```python
from build123d import *

# Parameters (mm, degrees)
F0_W     = 66.04
F0_H     = 22
F1_DEPTH = 69.85
F2_R     = 5.08


with BuildPart() as f1:
    # F0 (on Top) → F1 (new body)
    with BuildSketch(Plane.XY):
        Rectangle(F0_W, F0_H)
        with BuildLine():
            ThreePointArc((-23.97354, 8.353052), (-14.017672, 7.055087), (-11.109783, -2.554711))
            ThreePointArc((-11.109783, -2.554711), (-10.464057, -8.085959), (-16.02646, -8.353052))
            ThreePointArc((-16.02646, -8.353052), (-25.982328, -7.055087), (-28.890217, 2.554711))
            ThreePointArc((-28.890217, 2.554711), (-29.535943, 8.085959), (-23.97354, 8.353052))
        make_face(mode=Mode.SUBTRACT)
        with BuildLine():
            ThreePointArc((3.97354, -8.353052), (-5.982328, -7.055087), (-8.890217, 2.554711))
            ThreePointArc((-8.890217, 2.554711), (-9.535943, 8.085959), (-3.97354, 8.353052))
            ThreePointArc((-3.97354, 8.353052), (5.982328, 7.055087), (8.890217, -2.554711))
            ThreePointArc((8.890217, -2.554711), (9.535943, -8.085959), (3.97354, -8.353052))
        make_face(mode=Mode.SUBTRACT)
        with BuildLine():
            ThreePointArc((16.02646, 8.353052), (25.982328, 7.055087), (28.890217, -2.554711))
            ThreePointArc((28.890217, -2.554711), (29.535943, -8.085959), (23.97354, -8.353052))
            ThreePointArc((23.97354, -8.353052), (14.017672, -7.055087), (11.109783, 2.554711))
            ThreePointArc((11.109783, 2.554711), (10.464057, 8.085959), (16.02646, 8.353052))
        make_face(mode=Mode.SUBTRACT)
    extrude(amount=F1_DEPTH)

    # F2
    f2_edges = [f1.edges().sort_by_distance(p)[0] for p in [
        (-33.02, 11, 34.925),
        (-33.02, -11, 34.925),
        (33.02, -11, 34.925),
        (33.02, 11, 34.925),
    ]]
    fillet(f2_edges, radius=F2_R)


solid = f1.part
```
CAD build for the part. Positions are in the model's coordinates, mm. Coordinates: 2 decimals unless noted, no trailing zeros. Order: outer loops, then holes, each group sorted by start corner. A loop starts at its lowest first (then second) coordinate and runs counter-clockwise, first axis right, second up. Notation, with made-up numbers: (59, 45.5) - (76, 45.5) arc R27 ccw to (76, 67.5) - close; hole circle Ø6 at (57, 11). An arc over 180 degrees is marked (long way). Use a Markdown table: item, result. Add a question column.
(1) Flat gauge pins, fed straight in: pin 1 (1.5 mm diameter, centred on y = 8, z = 60, fed in from -X); pin 2 (5 mm diameter, centred on x = -18, y = 6, fed in from -Z). Where does each tip first touch, or does it go through?
(2) Saw through at A-A (x = -19). Give the cut face in (y, z), then the cut area to 3 significant figures.
(3) Saw through at C-C (z = 35). Give the cut face in (x, y).
(4) Drill centre lines: line 1 along X through (y, z) = (0.5, 61); line 2 along X through (y, z) = (2.75, 60); line 3 along Y through (x, z) = (-20.5, 19). Where is each one in solid material? Low to high. Write a range as [from, to].
(5) Pull direction Y, two halves, no side cores. Call faces 1 (the face through (33.02, 0, 34)), 2 (the face through (31.492, 9.551, 35.414)), 3 (the face through (-29.59, 8.02, 34.44)): +Y half, -Y half, draft (parallel to the pull), parting line (faces both ways), or undercut.
(6) Saw through at D-D (x = 26). Give the cut face in (y, z), then the cut area to 3 significant figures.
(7) Saw through at B-B (y = -7.25). Give the cut face in (x, z), then the cut area to 3 significant figures.
Solved:
| question | item | result |
|---|---|---|
| 1 | pin 1 | stops at x = -32.84 |
| 1 | pin 2 | passes through |
| 2 | outline | (-11, 0) - (-9.2, 0) - (-9.2, 69.85) - (-11, 69.85) - close; (9.2, 0) - (11, 0) - (11, 69.85) - (9.2, 69.85) - close |
| 2 | area | 252 mm² |
| 3 | outline | (-33.02, -5.92) arc R5.08 ccw to (-27.94, -11) - (27.94, -11) arc R5.08 ccw to (33.02, -5.92) - (33.02, 5.92) arc R5.08 ccw to (27.94, 11) - (-27.94, 11) arc R5.08 ccw to (-33.02, 5.92) - close; hole (-28.89, 2.55) arc R9.25 ccw to (-16.03, -8.35) arc R3.81 ccw (long way) to (-11.11, -2.55) arc R9.25 ccw to (-23.97, 8.35) arc R3.81 ccw (long way) to start; hole (-8.89, 2.55) arc R9.25 ccw to (3.97, -8.35) arc R3.81 ccw (long way) to (8.89, -2.55) arc R9.25 ccw to (-3.97, 8.35) arc R3.81 ccw (long way) to start; hole (11.11, 2.55) arc R9.25 ccw to (23.97, -8.35) arc R3.81 ccw (long way) to (28.89, -2.55) arc R9.25 ccw to (16.03, 8.35) arc R3.81 ccw (long way) to start |
| 4 | line 1 | x = [-33.02, -29.24], [-10.76, -9.24], [9.24, 10.76], [29.24, 33.02] |
| 4 | line 2 | x = [-33.02, -29.13], [-11.17, -9.13], [8.83, 10.87], [28.83, 33.02] |
| 4 | line 3 | y = [-11, -9.24], [9.24, 11] |
| 5 | face 1 | draft |
| 5 | face 2 | +Y half |
| 5 | face 3 | undercut |
| 6 | outline | (-11, 0) - (-9.38, 0) - (-9.38, 69.85) - (-11, 69.85) - close; (7.04, 0) - (11, 0) - (11, 69.85) - (7.04, 69.85) - close |
| 6 | area | 390 mm² |
| 7 | outline | (-32.84, 0) - (-25.74, 0) - (-25.74, 69.85) - (-32.84, 69.85) - close; (-9.93, 0) - (-5.74, 0) - (-5.74, 69.85) - (-9.93, 69.85) - close; (10.07, 0) - (14.26, 0) - (14.26, 69.85) - (10.07, 69.85) - close; (30.07, 0) - (32.84, 0) - (32.84, 69.85) - (30.07, 69.85) - close |
| 7 | area | 1,270 mm² |
